Source: CAD feature listing. Evaluate the final solid. Frame: model axes, mm. Coordinates: 2 decimals unless noted, no trailing zeros. Order: outer loops, then holes, each group sorted by start corner. A loop starts at its lowest first (then second) coordinate and runs counter-clockwise, first axis right, second up.
Item 1: Section A-A on x = 71.5. Return the cut outline in (y, z), then the cut area to 3 significant figures.
Item 2: Mould query, pull axis Y, two halves, no side actions, for faces 1 (the cylindrical face through (74.753, -1.232, -0.122)), 2 (the flat face through (77.342, 0, 0)), 3 (the flat face through (74.046, 5.655, 0.122)), 4 (the flat face through (74.14, -5.6, 0.12)). Classes: released by +Y, released by -Y, zero draft, split by the parting line, or undercut.
Item 3: Section D-D on y = -5. Return the cut outline in (x, z), then the cut area to 3 significant figures.
Item 4: Section B-B on z = 2. Return the cut outline in (x, y).
Item 5: Ray query, line 1 (Y direction, x = 71.25, z = 3.5); line 2 (Y direction, x = 70, z = 5.75); line 3 (X direction, y = 1.75, z = 2.5). Return the intervals inside material, ascending.
Item 6: Section C-C on y = 1.5. Return the cut outline in (x, z).
Item 7: Contact query for flat-ended pins moving along their axis: P1, Ø4, axis at y = 4, z = -3.5, coming from the +X side; P2, Ø5, axis at x = 66, z = -5, coming from the -Y side; P3, Ø1, axis at x = 66.5, z = 1, coming from the -Y side; P4, Ø5, axis at x = 70.84, y = 0, coming from the +Z side. Output: stop coordinate, or through.
Autodesk Inventor part; units mm, degrees
ref_plane "YZ Plane" through (0, 0, 0) normal (1, 0, 0) x (0, 1, 0)
ref_plane "XZ Plane" through (0, 0, 0) normal (0, 1, 0) x (-1, 0, 0)
ref_plane "XY Plane" through (0, 0, 0) normal (0, 0, 1) x (1, 0, 0)
sketch "Skizze1" plane through (0, 0, 0) normal (0, 0, 1) x (1, 0, 0)
  line L0 (70.8419, 7.621) -> (77.4419, 3.8105) construction
  line L1 (64.2419, 3.8105) -> (70.8419, 7.621) construction
  line L2 (70.8419, 7.5056) -> (77.3419, 3.7528)
  line L3 (77.3419, 3.7528) -> (77.3419, -3.7528)
  line L4 (77.3419, -3.7528) -> (70.8419, -7.5056)
  line L5 (70.8419, -7.5056) -> (64.3419, -3.7528)
  line L6 (64.3419, -3.7528) -> (64.3419, 3.7528)
  line L7 (64.3419, 3.7528) -> (70.8419, 7.5056)
  circle A0 centre (70.8419, 0) radius 4.1
  point P0 (0, 0)
  dimension "d0" = 13
  dimension "d1" = 8.2
extrude "Extrusion1" add sketch "Skizze1" against normal blind 8.7
mirror "Spiegeln1" about plane through (70.8419, 0, 0) normal (0, 0, 1) of "Extrusion1"
properties part number "Nutplacer" material "ABS-Kunststoff - Schwarz"
Answer list:
1. outline: (-7.13, -8.7) - (-4.05, -8.7) - (-4.05, 8.7) - (-7.13, 8.7) - close; (4.05, -8.7) - (7.13, -8.7) - (7.13, 8.7) - (4.05, 8.7) - close
1. area: 107 mm2
2. face 1: undercut
2. face 2: zero draft
2. face 3: released by +Y
2. face 4: released by -Y
3. outline: (66.5, -8.7) - (75.18, -8.7) - (75.18, 8.7) - (66.5, 8.7) - close
3. area: 151 mm2
4. outline: (64.34, -3.75) - (70.84, -7.51) - (77.34, -3.75) - (77.34, 3.75) - (70.84, 7.51) - (64.34, 3.75) - close; hole circle Ø8.2 at (70.84, 0)
5. line 1: y = -7.27 to -4.08, 4.08 to 7.27
5. line 2: y = -7.02 to -4.01, 4.01 to 7.02
5. line 3: x = 64.34 to 67.13, 74.55 to 77.34
6. outline: (64.34, -8.7) - (67.03, -8.7) - (67.03, 8.7) - (64.34, 8.7) - close; (74.66, -8.7) - (77.34, -8.7) - (77.34, 8.7) - (74.66, 8.7) - close
7. P1: stops at x = 77.34
7. P2: stops at y = -6.15
7. P3: stops at y = -5.29
7. P4: passes through
